Can you work these out from the model? Positions are in its coordinate system, mm. A direction names the side the tool comes from. Round coordinates to 2 decimals unless told otherwise and drop trailing zeros. Loops run counter-clockwise (first coordinate to the right, second up) from the corner with the lowest first, then second, coordinate; pieces in that order, holes last.
```python
from build123d import *

# Parameters (mm, degrees)
SKETCH1_W                      = 61.6
SKETCH1_H                      = 73.3
BOSS_EXTRUDE1_DEPTH            = 15.5
SKETCH2_W                      = 58.544
SKETCH2_H                      = 70.244
BOSS_EXTRUDE2_DEPTH            = 1
CUT_EXTRUDE1_DEPTH             = 1
CUT_EXTRUDE2_DEPTH             = 5.5
CUT_EXTRUDE3_DEPTH             = 8
SKETCH6_W                      = 1.1
SKETCH6_H                      = 18.4
CUT_EXTRUDE4_DEPTH             = 9.3
SKETCH7_W                      = 1.1
SKETCH7_H                      = 18.4
CUT_EXTRUDE5_DEPTH             = 9.3
F_2_2_2_2_DIAMETER_HOLE1_D     = 2.2
F_2_2_2_2_DIAMETER_HOLE1_DEPTH = 7.6
FILLET1_R                      = 2
FILLET2_R                      = 4.871984114
FILLET3_R                      = 5.472
FILLET4_R                      = 7


with BuildPart() as part:
    # Sketch1 → Boss-Extrude1 (new body)
    with BuildSketch(Plane(origin=(0, 0, 0.5), x_dir=(-1, 0, 0), z_dir=(0, 0, -1))):
        with Locations((-23.1, -18.15)):
            Rectangle(SKETCH1_W, SKETCH1_H)
    extrude(amount=-BOSS_EXTRUDE1_DEPTH)

    # Sketch2 → Boss-Extrude2 (add)
    with BuildSketch(Plane(origin=(0, 0, 0.5), x_dir=(-1, 0, 0), z_dir=(0, 0, -1))):
        with Locations((-23.1, -18.15)):
            Rectangle(SKETCH2_W, SKETCH2_H)
    extrude(amount=BOSS_EXTRUDE2_DEPTH)

    # Sketch3 → Cut-Extrude1 (cut)
    with BuildSketch(Plane(origin=(0, 0, -0.5), x_dir=(-1, 0, 0), z_dir=(0, 0, -1))):
        with BuildLine():
            Line((-51.771984114, 16.371984114), (-51.771984114, -35.734235116))
            Line((-51.771984114, -35.734235116), (-49.52987247, -35.734235116))
            Line((-49.52987247, -35.734235116), (-49.52987247, -51.901219331))
            ThreePointArc((-49.52987247, -51.901219331), (-48.270247018, -52.475323766), (-46.9, -52.671984114))
            Line((-46.9, -52.671984114), (0.7, -52.671984114))
            ThreePointArc((0.7, -52.671984114), (2.070247018, -52.475323766), (3.32987247, -51.901219331))
            Line((3.32987247, -51.901219331), (3.32987247, -35.734235116))
            Line((3.32987247, -35.734235116), (5.571984114, -35.734235116))
            Line((5.571984114, -35.734235116), (5.571984114, 16.371984114))
            Line((5.571984114, 16.371984114), (-51.771984114, 16.371984114))
        make_face()
    extrude(amount=-CUT_EXTRUDE1_DEPTH, mode=Mode.SUBTRACT)

    # Sketch4 → Cut-Extrude2 (cut)
    with BuildSketch(Plane(origin=(0, 0, 0.5), x_dir=(-1, 0, 0), z_dir=(0, 0, -1))):
        Polygon((3, -14.8), (4.7, -14.8), (4.7, 15.5), (-50.9, 15.5), (-50.9, -14.8), (-49.2, -14.8), (-49.2, -31.8), (-45.2, -31.8), (-45.2, -50.2), (-1, -50.2), (-1, -31.8), (3, -31.8), align=None)
    extrude(amount=-CUT_EXTRUDE2_DEPTH, mode=Mode.SUBTRACT)

    # Sketch5 → Cut-Extrude3 (cut)
    with BuildSketch(Plane(origin=(0, 0, 6), x_dir=(-1, 0, 0), z_dir=(0, 0, -1))):
        Polygon((3, -12.7), (-1, -12.7), (-1, -11.5), (4.7, -11.5), (4.7, 15.5), (-50.9, 15.5), (-50.9, -11.5), (-45.2, -11.5), (-45.2, -12.7), (-49.2, -12.7), (-49.2, -31.8), (-45.2, -31.8), (-45.2, -50.2), (-1, -50.2), (-1, -31.8), (3, -31.8), align=None)
    extrude(amount=-CUT_EXTRUDE3_DEPTH, mode=Mode.SUBTRACT)

    # Sketch6 → Cut-Extrude4 (cut)
    with BuildSketch(Plane(origin=(0, 0, 0.5), x_dir=(-1, 0, 0), z_dir=(0, 0, -1))):
        with Locations((-45.75, -41)):
            Rectangle(SKETCH6_W, SKETCH6_H)
    extrude(amount=-CUT_EXTRUDE4_DEPTH, mode=Mode.SUBTRACT)

    # Sketch7 → Cut-Extrude5 (cut)
    with BuildSketch(Plane(origin=(0, 0, 0.5), x_dir=(-1, 0, 0), z_dir=(0, 0, -1))):
        with Locations((-0.45, -41)):
            Rectangle(SKETCH7_W, SKETCH7_H)
    extrude(amount=-CUT_EXTRUDE5_DEPTH, mode=Mode.SUBTRACT)

    # Ø2.2 (2.2) Diameter Hole1
    with Locations(Plane(origin=(-0.1, 0, 0), x_dir=(0, 0, -1), z_dir=(1, 0, 0))):
        with Locations((-5, -41.2)):
            Hole(F_2_2_2_2_DIAMETER_HOLE1_D / 2, depth=F_2_2_2_2_DIAMETER_HOLE1_DEPTH)

    # Fillet1
    fillet1_edges = [part.edges().sort_by_distance(p)[0] for p in [
        (23.1, -54.8, 16),
        (-7.7, -18.15, 16),
        (23.1, 18.5, 16),
        (50.9, 15.5, 7.25),
        (-4.7, 15.5, 7.25),
        (53.9, -18.15, 16),
    ]]
    fillet(fillet1_edges, radius=FILLET1_R)

    # Fillet2
    fillet2_edges = [part.edges().sort_by_distance(p)[0] for p in [
        (51.771984114, 16.371984114, 0),
        (-5.571984114, 16.371984114, 0),
    ]]
    fillet(fillet2_edges, radius=FILLET2_R)

    # Fillet3
    fillet3_edges = [part.edges().sort_by_distance(p)[0] for p in [
        (52.372, 16.972, 0),
        (52.372, -53.272, 0),
        (-6.172, -53.272, 0),
        (-6.172, 16.972, 0),
    ]]
    fillet(fillet3_edges, radius=FILLET3_R)

    # Fillet4
    # the kernel refuses this fillet: 7 mm, written as the material it takes off along each edge
    with BuildSketch(Plane(origin=(-7.7, -54.8, -17), x_dir=(1, 0, 0), z_dir=(0, 0, 1)), Plane(origin=(53.9, -54.8, -17), x_dir=(0, 1, 0), z_dir=(0, 0, 1))) as fillet4_piece_1:
        with BuildLine():
            CenterArc((FILLET4_R, FILLET4_R), FILLET4_R, 180, 90)
            Line((0, FILLET4_R), (0, 0))
            Line((0, 0), (FILLET4_R, 0))
        make_face()
    extrude(amount=48.5, mode=Mode.SUBTRACT)
    with BuildSketch(Plane(origin=(-7.7, 18.5, -17), x_dir=(1, 0, 0), z_dir=(0, 0, 1)), Plane(origin=(53.9, 18.5, -17), x_dir=(0, -1, 0), z_dir=(0, 0, 1))) as fillet4_piece_2:
        with BuildLine():
            CenterArc((FILLET4_R, -FILLET4_R), FILLET4_R, 90, 90)
            Line((0, -FILLET4_R), (0, 0))
            Line((0, 0), (FILLET4_R, 0))
        make_face()
    extrude(amount=48.5, mode=Mode.SUBTRACT)


solid = part.part
```
(1) Suppose I cut it at C-C (x = 39.5). Write out the boundary of the cut face in (y, z).
(2) Suppose I cut it at B-B (y = 6.5). Write out the boundary of the cut face in (x, z).
(3) We'd pull the mould along X, two halves only. Please class faces 5 (the flat face through (-4.7, -1, 7)), 6 (the cylindrical face through (-4.53, -51.71, -0.01)), 7 (the flat face through (51, -39, -0.5)), 8 (the flat face through (53.9, -19, 7)): released by +X, released by -X, zero draft, split by the parting line, or undercut.
(4) If I drill on line 1 (X direction, y = 5.5, z = 4); line 2 (Y direction, x = 3, z = 9); line 3 (X direction, y = -34, z = 8.75), over which ranges is the centre line in solid material (lowest first)?
(5) Suppose I cut it at A-A (y = -41.2). Write out the boundary of the cut face in (x, z).
(6) Which directions (+Z, -Z, +X, -X, +Y, -Y) give clear straight access to the entire face, cutting with the end or side of a thin tool? Please do faces 1 (the cylindrical face through (51.9, 16.4, 8.1)), 2 (the flat face through (50, -14.8, 3)), 3 (the cylindrical face through (50.81, -51.63, -0.01)), 4 (the cylindrical face through (50.81, 15.33, -0.01)).
(7) For pin 1 (5 mm diameter, centred on x = 13.5, y = 0.5, fed in from -Z); pin 2 (0.9 mm diameter, centred on x = 0.5, y = -39, fed in from -Z); pin 3 (0.5 mm diameter, centred on x = 29, z = 0, fed in from -Y), each with a flat end and sliding along its axis, tell me the tip position at first contact or that it passes through.
(8) Suppose I cut it at D-D (z = 5). Write out the boundary of the cut face in (x, y).
Check result:
1. outline: (-54.8, 0.5) - (-53.27, 0.5) - (-53.27, -0.5) - (-52.67, -0.5) - (-52.67, 0.5) - (-50.2, 0.5) - (-50.2, 14) - (15.5, 14) - (15.5, 0.5) - (16.37, 0.5) - (16.37, -0.5) - (16.97, -0.5) - (16.97, 0.5) - (18.5, 0.5) - (18.5, 14) arc R2 ccw to (16.5, 16) - (-52.8, 16) arc R2 ccw to (-54.8, 14) - close
2. outline: (-7.7, 0.5) - (-6.17, 0.5) - (-6.17, -0.5) - (-5.57, -0.5) - (-5.57, 0.5) - (-4.7, 0.5) - (-4.7, 14) - (50.9, 14) - (50.9, 0.5) - (51.77, 0.5) - (51.77, -0.5) - (52.37, -0.5) - (52.37, 0.5) - (53.9, 0.5) - (53.9, 14) arc R2 ccw to (51.9, 16) - (-5.7, 16) arc R2 ccw to (-7.7, 14) - close
3. face 5: undercut
3. face 6: released by -X
3. face 7: zero draft
3. face 8: released by +X
4. line 1: x = -7.7 to -4.7, 50.9 to 53.9
4. line 2: y = -54.8 to -50.2, 15.5 to 18.5
4. line 3: x = -7.7 to -0.1, 46.3 to 53.9
5. outline: (-7.7, 0.5) - (-6.17, 0.5) - (-6.17, -0.5) - (-3.33, -0.5) - (-3.33, 0.5) - (-0.1, 0.5) - (-0.1, 3.9) - (-7.7, 3.9) - close; (-7.7, 6.1) - (-0.1, 6.1) - (-0.1, 9.8) - (1, 9.8) - (1, 14) - (45.2, 14) - (45.2, 9.8) - (46.3, 9.8) - (46.3, 0.5) - (49.53, 0.5) - (49.53, -0.5) - (52.37, -0.5) - (52.37, 0.5) - (53.9, 0.5) - (53.9, 14) arc R2 ccw to (51.9, 16) - (-5.7, 16) arc R2 ccw to (-7.7, 14) - close
6. face 1: +Z, -Z, +X, +Y
6. face 2: -Z
6. face 3: -Z, +X, -Y
6. face 4: -Z, +X, +Y
7. pin 1: stops at z = 14
7. pin 2: stops at z = 9.8
7. pin 3: stops at y = -53.27
8. outline: (-7.7, -47.8) arc R7 ccw to (-0.7, -54.8) - (46.9, -54.8) arc R7 ccw to (53.9, -47.8) - (53.9, 11.5) arc R7 ccw to (46.9, 18.5) - (-0.7, 18.5) arc R7 ccw to (-7.7, 11.5) - (-7.7, -40.1) - (-0.1, -40.1) - (-0.1, -31.8) - (-3, -31.8) - (-3, -14.8) - (-4.7, -14.8) - (-4.7, 13.5) arc R2 cw to (-2.7, 15.5) - (48.9, 15.5) arc R2 cw to (50.9, 13.5) - (50.9, -14.8) - (49.2, -14.8) - (49.2, -31.8) - (46.3, -31.8) - (46.3, -50.2) - (-0.1, -50.2) - (-0.1, -42.3) - (-7.7, -42.3) - close
